from build123d import *

# Parameters (mm, degrees)
SKETCH1_R           = 1
BOSS_EXTRUDE1_DEPTH = 8
FILLET1_R           = 1


with BuildPart() as part:
    # Sketch1 → Boss-Extrude1 (new body)
    with BuildSketch(Plane.XY):
        Polygon((0, 0), (0, 10), (8, 10), (8, 48.5), (-10, 48.5), (-10, 40.5), (2, 40.5), (2, 18), (-10, 18), (-10, 10), (-10, 0), align=None)
        with Locations((-4, 43.1)):
            Circle(SKETCH1_R, mode=Mode.SUBTRACT)
        with Locations((-4, 15.4)):
            Circle(SKETCH1_R, mode=Mode.SUBTRACT)
    extrude(amount=BOSS_EXTRUDE1_DEPTH)

    # Fillet1
    fillet1_edges = [part.edges().sort_by_distance(p)[0] for p in [
        (-10, 18, 4),
        (-10, 40.5, 4),
        (-10, 48.5, 4),
        (8, 48.5, 4),
        (8, 10, 4),
    ]]
    fillet(fillet1_edges, radius=FILLET1_R)


solid = part.part
Here's how the part is built. I have some questions about the finished solid (model axes, mm). A direction names the side the tool comes from. Round coordinates to 2 decimals unless told otherwise and drop trailing zeros. Loops run counter-clockwise (first coordinate to the right, second up) from the corner with the lowest first, then second, coordinate; pieces in that order, holes last. Notation, with made-up numbers: (72, 77) -> (114, 77) arc R22 ccw to (114, 106) -> close; hole circle Ø1 at (59, -6). An arc over 180 degrees is marked (long way). Write each question's results on one line, items separated by ' | '.
(1) If we section it at A-A, the plane y = 43.1: List the corners of the cut face in (x, z) for me.
Worked answers:
outline: (-10, 0) -> (-5, 0) -> (-5, 8) -> (-10, 8) -> close; (-3, 0) -> (8, 0) -> (8, 8) -> (-3, 8) -> close
(2) If we section it at B-B, the plane x = -1.5: List the corners of the cut face in (y, z) for me, then the cut area to 3 significant figures.
Worked answers:
outline: (0, 0) -> (18, 0) -> (18, 8) -> (0, 8) -> close; (40.5, 0) -> (48.5, 0) -> (48.5, 8) -> (40.5, 8) -> close | area: 208 mm2
(3) We'd pull the mould along Y, two halves only. Please class faces 1 (the face through (-4.13, 44.09, 3.94)), 2 (the face through (3, 25, 0)), 3 (the face through (7.699, 10.285, 4.056)), 4 (the face through (-4, 40.5, 4)): released by +Y, released by -Y, zero draft, split by the parting line, or undercut.
Worked answers:
face 1: undercut | face 2: zero draft | face 3: released by -Y | face 4: undercut
(4) For faces 5 (the face through (0, 5, 4)), 6 (the face through (2, 29, 4)), 7 (the face through (-5, 0, 4)), which set-ups out of +Z, -Z, +X, -X, +Y, -Y let a thin tool reach every point of the face, with its end or its side?
Worked answers:
face 5: +Z, -Z, +X, -Y | face 6: +Z, -Z, -X | face 7: +Z, -Z, +X, -X, -Y
(5) If we section it at C-C, the plane z = 6.5: List the corners of the cut face in (x, y) for me.
Worked answers:
outline: (-10, 0) -> (0, 0) -> (0, 10) -> (7, 10) arc R1 ccw to (8, 11) -> (8, 47.5) arc R1 ccw to (7, 48.5) -> (-9, 48.5) arc R1 ccw to (-10, 47.5) -> (-10, 41.5) arc R1 ccw to (-9, 40.5) -> (2, 40.5) -> (2, 18) -> (-9, 18) arc R1 ccw to (-10, 17) -> close; hole circle Ø2 at (-4, 15.4); hole circle Ø2 at (-4, 43.1)
(6) If I drill on L1, parallel to Y at x = -4, z = 2; L2, parallel to Y at x = -1, z = 2.25; L3, parallel to Y at x = 0.75, z = 3, over which ranges is the centre line in solid material (lowest first)?
Worked answers:
L1: 0 to 14.4, 16.4 to 18, 40.5 to 42.1, 44.1 to 48.5 | L2: 0 to 18, 40.5 to 48.5 | L3: 10 to 18, 40.5 to 48.5
(7) If we section it at D-D, the plane x = -4: List the corners of the cut face in (y, z) for me, then the cut area to 3 significant figures.
Worked answers:
outline: (0, 0) -> (14.4, 0) -> (14.4, 8) -> (0, 8) -> close; (16.4, 0) -> (18, 0) -> (18, 8) -> (16.4, 8) -> close; (40.5, 0) -> (42.1, 0) -> (42.1, 8) -> (40.5, 8) -> close; (44.1, 0) -> (48.5, 0) -> (48.5, 8) -> (44.1, 8) -> close | area: 176 mm2
(8) For P1, Ø3, axis at y = 29.5, z = 1, coming from the -X side; P2, Ø2, axis at x = 5, z = 4, coming from the -Y side; P3, Ø2.5, axis at y = 7, z = 3, coming from the +X side, each with a flat end and sliding along its axis, tell me the tip position at first contact or that it passes through.
Worked answers:
P1: x = 2 | P2: y = 10 | P3: x = 0
